The listing builds one solid part. Answer for the finished solid, in the listing's coordinates (mm). A direction names the side the tool comes from. Round coordinates to 2 decimals unless told otherwise and drop trailing zeros. Loops run counter-clockwise (first coordinate to the right, second up) from the corner with the lowest first, then second, coordinate; pieces in that order, holes last. Notation, with made-up numbers: M 75.5,79 L 90.5,79 A31 cw 90.5,114 Z; hole C 75,-17 d5. An arc over 180 degrees is marked long. Answer as a JSON object with one key per item and string values.
```python
from build123d import *

# Parameters (mm, degrees)
CROQUIS1_R              = 5
SALIENTE_EXTRUIR1_DEPTH = 5
CROQUIS2_R              = 7
SALIENTE_EXTRUIR2_DEPTH = 3
CROQUIS3_R              = 14
SALIENTE_EXTRUIR3_DEPTH = 3
CROQUIS4_R              = 6
SALIENTE_EXTRUIR4_DEPTH = 24
CROQUIS5_R              = 5
SALIENTE_EXTRUIR5_DEPTH = 5
CROQUIS6_R              = 1.5
CORTAR_EXTRUIR1_DEPTH   = 5
CHAFL_N1_SIZE           = 1.5


with BuildPart() as part:
    # Croquis1 → Saliente-Extruir1 (new body)
    with BuildSketch(Plane.XY):
        Circle(CROQUIS1_R)
    extrude(amount=SALIENTE_EXTRUIR1_DEPTH)

    # Croquis2 → Saliente-Extruir2 (add)
    with BuildSketch(Plane.XY.offset(5)):
        Circle(CROQUIS2_R)
    extrude(amount=SALIENTE_EXTRUIR2_DEPTH)

    # Croquis3 → Saliente-Extruir3 (add)
    with BuildSketch(Plane.XY.offset(8)):
        Circle(CROQUIS3_R)
    extrude(amount=SALIENTE_EXTRUIR3_DEPTH)

    # Croquis4 → Saliente-Extruir4 (add)
    with BuildSketch(Plane.XY.offset(11)):
        Circle(CROQUIS4_R)
    extrude(amount=SALIENTE_EXTRUIR4_DEPTH)

    # Croquis5 → Saliente-Extruir5 (add)
    with BuildSketch(Plane.XY.offset(35)):
        Circle(CROQUIS5_R)
    extrude(amount=SALIENTE_EXTRUIR5_DEPTH)

    # Croquis6 → Cortar-Extruir1 (cut)
    with BuildSketch(Plane(origin=(0, 0, 8), x_dir=(-1, 0, 0), z_dir=(0, 0, -1))):
        with Locations((11, 0)):
            Circle(CROQUIS6_R)
        with Locations((0, -11)):
            Circle(CROQUIS6_R)
        with Locations((-11, 0)):
            Circle(CROQUIS6_R)
        with Locations((0, 11)):
            Circle(CROQUIS6_R)
    extrude(amount=-CORTAR_EXTRUIR1_DEPTH, mode=Mode.SUBTRACT)

    # Chaflán1
    chafl_n1_edges = [part.edges().sort_by_distance(p)[0] for p in [
        (-9.5, 0, 8),
        (1.5, -11, 8),
        (12.5, 0, 8),
        (1.5, 11, 8),
    ]]
    chamfer(chafl_n1_edges, length=CHAFL_N1_SIZE - 0.0001)  # a hair under: the kernel refuses the full size


solid = part.part
```
Item 1: Which of the six approach directions +Z, -Z, +X, -X, +Y, -Y give full straight-line access (tool end or side, diameter ignored) to faces 5 (the face through (-6, 0, 23)), 6 (the face through (-6.4, 3.3, 8)), 7 (the face through (-9.5, 0.07, 10.24))?
Values follow:
{"face 5": "+Z", "face 6": "-Z", "face 7": "+Z, -Z"}
Item 2: Flat-ended cylindrical pins translate along their axes: P1, Ø4, axis at x = -11, y = 0, coming from the -Z side; P2, Ø3.5, axis at x = 0, y = 11, coming from the -Z side; P3, Ø2.5, axis at x = 0, y = -11, coming from the -Z side; P4, Ø8, axis at x = 0, z = 29, coming from the -Y side. Find the tip coordinate at first contact, or state that the pin passes through.
Values follow:
{"P1": "z = 9", "P2": "z = 9.25", "P3": "through", "P4": "y = -6"}
Item 3: The part is cut by section A-A (y = 0). Give the number of separate pieces and of enclosed holes in the cut face, then the cut area to 4 significant figures.
Values follow:
{"separate pieces": "3", "enclosed holes": "0", "area": "491.5 mm^2"}
Item 4: Determine the mould class of faces 1 (the face through (-9, 0, 9)), 2 (the face through (13, 0, 9)), 3 (the face through (-1.08, -4.88, 2.46)), 4 (the face through (-4, 4, 35)) for opening direction Y: released by +Y, released by -Y, zero draft, split by the parting line, or undercut.
Values follow:
{"face 1": "undercut", "face 2": "undercut", "face 3": "split by the parting line", "face 4": "zero draft"}
Item 5: Straight lines are drawn through the part: line 1 (Y direction, x = 0, z = 10.4); line 2 (Z direction, x = 6, y = 3); line 3 (Z direction, x = -4, y = -12). For each, find the intervals that lie inside material, in ascending order.
Values follow:
{"line 1": "-14 to -12.5, -9.5 to 9.5, 12.5 to 14", "line 2": "5 to 11", "line 3": "8 to 11"}
Item 6: The part is cut by section B-B (x = -11). Give the vertices of the cut face in (y, z).
Values follow:
{"outline": "M -8.66,8 L -3,8 L -1.5,9.5 L -1.5,11 L -8.66,11 Z; M 1.5,9.5 L 3,8 L 8.66,8 L 8.66,11 L 1.5,11 Z"}
Item 7: The part is cut by section D-D (z = 36). Give the vertices of the cut face in (x, y), then the cut area to 3 significant figures.
Values follow:
{"outline": "C 0,0 d10", "area": "78.5 mm^2"}
